Could you check a few things on this drawing? It's one solid part, dimensions in mm from its lowest x, y, z. A direction names the side the tool comes from. Give positions to 0.01 mm unless a question says otherwise; leave off trailing zeros. Write each loop counter-clockwise with the first axis right and the second up, starting at its lowest first coordinate (ties: lowest second). Pieces come first, ordered by that corner, then holes. Notation, with made-up numbers: (23.25, -31) -> (59.25, -31) arc R6 cw to (59.25, -26) -> close; hole circle Ø6 at (-32, -37). An arc over 180 degrees is marked (long way). Use CSV: the item, a comma, the result in double quotes. Start each with the question number.
(1) Suppose I cut it at B-B on x = 23.5. List the corners of the cut face in (y, z) for me (1 decimal).
(2) For pin 1 Ø12.5 at (x, y) = (17.5, 15) entering from -Z; pin 2 Ø11 at (x, z) = (23.5, 20.5) entering from -Y (1 decimal), each with a flat end and sliding along its axis, tell me the tip position at first contact or that it passes through.
(3) Suppose I cut it at D-D on z = 12. List the corners of the cut face in (x, y) for me (1 decimal), plus the area to 3 significant figures.
(4) Suppose I cut it at C-C on z = 19. List the corners of the cut face in (x, y) for me (1 decimal).
(5) Which directions (+Z, -Z, +X, -X, +Y, -Y) give clear straight access to the entire face, cutting with the end or side of a thin tool? Please do the marked faces 1 and 2.
(6) I need wall thicknesses on L1, parallel to X at y = 6.5, z = 21 (1 decimal); L2, parallel to Z at x = 14, y = 4 (1 decimal); L3, parallel to Y at x = 27.5, z = 7.5 (1 decimal). Which ranges of each line are inside material? Lowest first, please. Write a range as [from, to].
(7) Suppose I cut it at A-A on y = 11. List the corners of the cut face in (x, z) for me (1 decimal), plus the area to 3 significant figures.
(8) If we mould it in two halves opening along X, with no side actions, what happens to the marked faces 3, 4 and 5? For each: pulls with the +X half, pulls with the -X half, needs draft (parallel to the pull), parting line crosses it, or undercut.
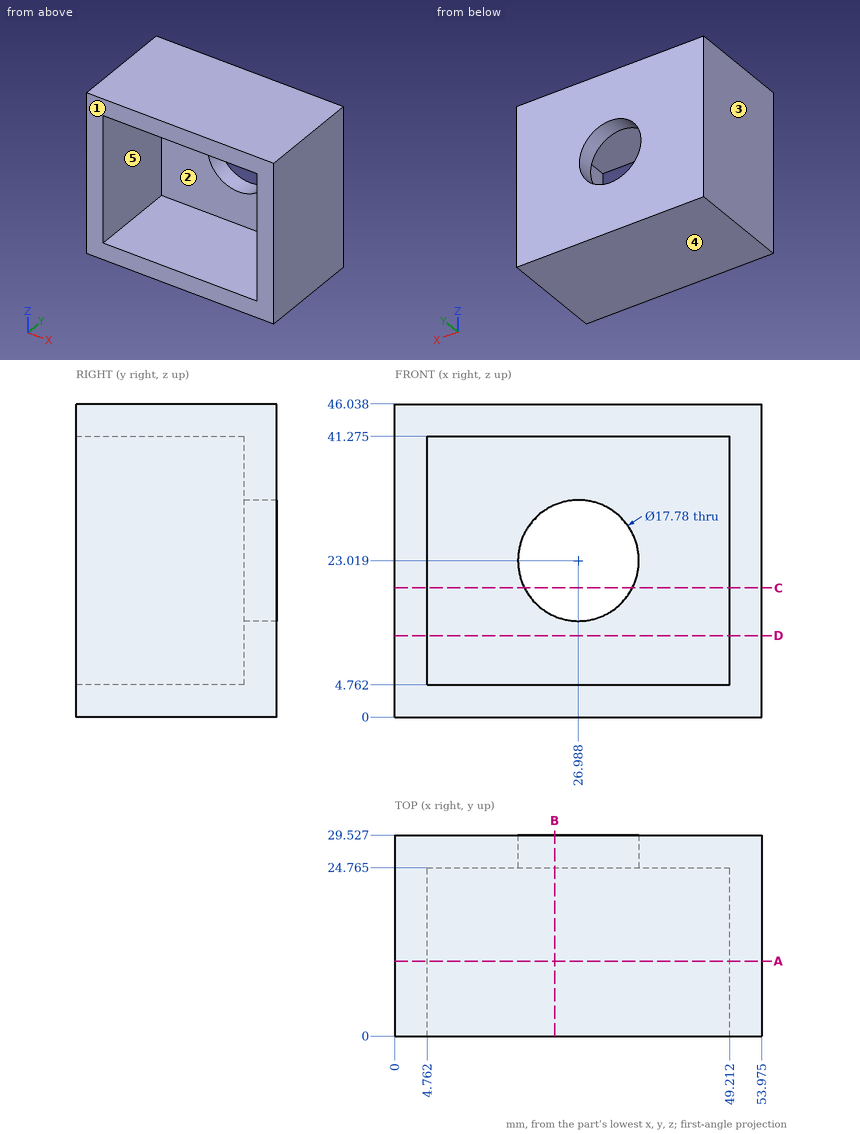
Geometry says:
1,outline,"(0, 0) -> (29.5, 0) -> (29.5, 14.8) -> (24.8, 14.8) -> (24.8, 4.8) -> (0, 4.8) -> close; (0, 41.3) -> (24.8, 41.3) -> (24.8, 31.2) -> (29.5, 31.2) -> (29.5, 46) -> (0, 46) -> close"
2,pin 1,"z = 0"
2,pin 2,"y = 24.8"
3,outline,"(0, 0) -> (4.8, 0) -> (4.8, 24.8) -> (49.2, 24.8) -> (49.2, 0) -> (54, 0) -> (54, 29.5) -> (0, 29.5) -> close"
3,area,"493 mm²"
4,outline,"(0, 0) -> (4.8, 0) -> (4.8, 24.8) -> (19.1, 24.8) -> (19.1, 29.5) -> (0, 29.5) -> close; (34.9, 24.8) -> (49.2, 24.8) -> (49.2, 0) -> (54, 0) -> (54, 29.5) -> (34.9, 29.5) -> close"
5,face 1,"+Z, -Z, +X, -X, -Y"
5,face 2,"-Y"
6,L1,"[0, 4.8], [49.2, 54]"
6,L2,"[0, 4.8], [41.3, 46]"
6,L3,"[24.8, 29.5]"
7,outline,"(0, 0) -> (54, 0) -> (54, 46) -> (0, 46) -> close; hole (4.8, 4.8) -> (49.2, 4.8) -> (49.2, 41.3) -> (4.8, 41.3) -> close"
7,area,"862 mm²"
8,face 3,"pulls with the -X half"
8,face 4,"needs draft"
8,face 5,"undercut"
